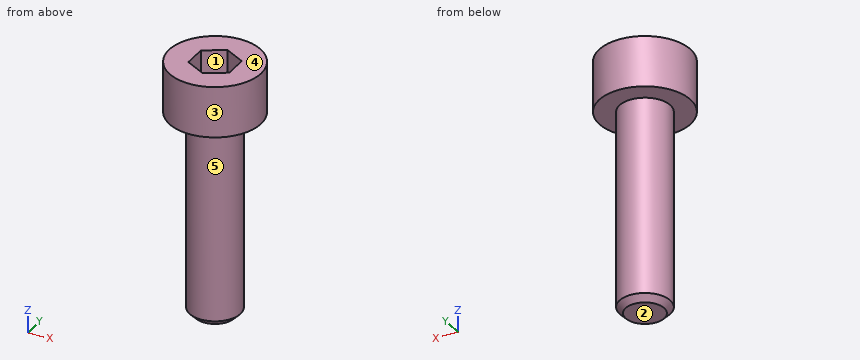
```python
from build123d import *

# Parameters (mm, degrees)
SKETCH1_R           = 2.25
BOSS_EXTRUDE1_DEPTH = 2.5
SKETCH2_R           = 1.25
BOSS_EXTRUDE2_DEPTH = 10
CHAMFER1_SIZE       = 0.3
CUT_EXTRUDE1_DEPTH  = 2


with BuildPart() as part:
    # Sketch1 → Boss-Extrude1 (new body)
    with BuildSketch(Plane.XY):
        Circle(SKETCH1_R)
    extrude(amount=BOSS_EXTRUDE1_DEPTH)

    # Sketch2 → Boss-Extrude2 (add)
    with BuildSketch(Plane(origin=(0, 0, 0), x_dir=(-1, 0, 0), z_dir=(0, 0, -1))):
        Circle(SKETCH2_R)
    extrude(amount=BOSS_EXTRUDE2_DEPTH)

    # Chamfer1
    chamfer1_edges = [part.edges().sort_by_distance(p)[0] for p in [
        (1.25, 0, -10),
    ]]
    chamfer(chamfer1_edges, length=CHAMFER1_SIZE)

    # Sketch3 → Cut-Extrude1 (cut)
    with BuildSketch(Plane.XY.offset(2.5)):
        Polygon((0, 1.154700538), (-1, 0.577350269), (-1, -0.577350269), (0, -1.154700538), (1, -0.577350269), (1, 0.577350269), align=None)
    extrude(amount=-CUT_EXTRUDE1_DEPTH, mode=Mode.SUBTRACT)


solid = part.part
```
Build history of the part. All positions in model axes, mm. Face numbers are marked on the shaded views. A direction names the side the tool comes from. Give positions to 0.01 mm unless a question says otherwise; leave off trailing zeros. Order: outer loops, then holes, each group sorted by start corner. A loop starts at its lowest first (then second) coordinate and runs counter-clockwise, first axis right, second up. Notation, with made-up numbers: M -31,46.5 L -13,46.5 A13 ccw -13,52.5 Z; hole C 60,-20 d11. An arc over 180 degrees is marked long. Write item = value, one per line. Start each with the question number.
(1) Which spindle directions (+Z, -Z, +X, -X, +Y, -Y) get a long thin tool onto all of the face, cutting with end or side? Do the marked faces 4 and 5. Say none if no direction does.
(2) Slice it at C-C on x = -1.7. Write the cut outline in (y, z), plus the area to 3 significant figures.
(3) Slice it at A-A on y = 0. Write the cut outline in (x, z).
(4) Slice it at D-D on y = 1.9. Write the cut outline in (x, z).
(5) Two-plate mould, pull along Y, no slides. Class the marked faces 1, 2 and 3: released by +Y, released by -Y, zero draft, split by the parting line, or undercut.
(6) Pin check, flat tips, straight feed: pin 1 Ø1.5 at (x, z) = (1, -3) entering from -Y; pin 2 Ø1.6 at (x, y) = (0, 0) entering from +Z. Stop position of each tip, or through.
(7) Slice it at B-B on z = -1.75. Write the cut outline in (x, y).
(8) Probe L1, parallel to X at y = 0.05, z = -1.25; L2, parallel to Z at x = -1.15, y = -1.2; L3, parallel to Z at x = 0.6, y = -0.4. List the from-to ranges inside material, lowest first. Write a range as [from, to].
Responses:
q1.face_4 = +Z, +X, -X, +Y, -Y
q1.face_5 = -Z
q2.outline = M -1.47,0 L 1.47,0 L 1.47,2.5 L -1.47,2.5 Z
q2.area = 7.37 mm2
q3.outline = M -2.25,0 L -1.25,0 L -1.25,-9.7 L -0.95,-10 L 0.95,-10 L 1.25,-9.7 L 1.25,0 L 2.25,0 L 2.25,2.5 L 1,2.5 L 1,0.5 L -1,0.5 L -1,2.5 L -2.25,2.5 Z
q4.outline = M -1.21,0 L 1.21,0 L 1.21,2.5 L -1.21,2.5 Z
q5.face_1 = undercut
q5.face_2 = zero draft
q5.face_3 = split by the parting line
q6.pin_1 = -1.22
q6.pin_2 = 0.5
q7.outline = C 0,0 d2.5
q8.L1 = [-1.25, 1.25]
q8.L2 = [0, 2.5]
q8.L3 = [-10, 0.5]
